Check sheet for the modelled part. Datum: model origin and axes. Units: mm. A direction names the side the tool comes from. Round coordinates to 2 decimals unless told otherwise and drop trailing zeros. Write each loop counter-clockwise with the first axis right and the second up, starting at its lowest first coordinate (ties: lowest second). Pieces come first, ordered by that corner, then holes.
from build123d import *

# Parameters (mm, degrees)
F0_R     = 3.96875
F1_DEPTH = 25.4
F2_R     = 1.524


with BuildPart() as f1:
    # F0 (on Front) → F1 (new body)
    with BuildSketch(Plane.XZ):
        with BuildLine():
            Line((0, 596.9), (0, 0))
            Line((0, 0), (25.4, 0))
            Line((25.4, 0), (25.4, 596.9))
            ThreePointArc((25.4, 596.9), (55.157951, 668.742049), (127, 698.5))
            Line((127, 698.5), (396.875, 698.5))
            Line((396.875, 698.5), (396.875, 723.9))
            Line((396.875, 723.9), (127, 723.9))
            ThreePointArc((127, 723.9), (37.197439, 686.702561), (0, 596.9))
        make_face()
        with Locations((12.7, 120.65)):
            Circle(F0_R, mode=Mode.SUBTRACT)
        with Locations((12.7, 215.9)):
            Circle(F0_R, mode=Mode.SUBTRACT)
    extrude(amount=F1_DEPTH)

    # F2
    f2_edges = [f1.edges().sort_by_distance(p)[0] for p in [
        (25.4, -25.4, 298.45),
        (0, -25.4, 298.45),
        (0, 0, 298.45),
        (25.4, 0, 298.45),
        (12.7, 0, 0),
        (55.157951, 0, 668.742049),
        (261.9375, 0, 698.5),
        (396.875, 0, 711.2),
        (261.9375, 0, 723.9),
        (37.197439, 0, 686.702561),
        (8.73125, 0, 120.65),
        (8.73125, 0, 215.9),
        (12.7, -25.4, 0),
        (55.157951, -25.4, 668.742049),
        (261.9375, -25.4, 698.5),
        (396.875, -25.4, 711.2),
        (261.9375, -25.4, 723.9),
        (37.197439, -25.4, 686.702561),
        (8.73125, -25.4, 120.65),
        (8.73125, -25.4, 215.9),
    ]]
    fillet(f2_edges, radius=F2_R)


solid = f1.part
1. Sectioned sample at C-C, the plane x = 251. Enter the section's corners in (y, z).
2. Set-up check for faces 4 (the cylindrical face through (38.19, -12.544, 687.685)), 5 (the flat face through (25.4, -13, 294)): record each of +Z, -Z, +X, -X, +Y, -Y from which the full face is reachable in a straight line by a thin tool's end or side.
3. Scan lines: line 1 along Z through (x, y) = (12.7, -14.25); line 2 along X through (y, z) = (-15.75, 509.5); line 3 along Z through (x, y) = (200.5, -19.75). Record each from-to range of solid material in increasing order.
4. Release check for a two-part mould opening along Y. For faces 1 (the flat face through (22, 0, 470)), 2 (the flat face through (264, -13, 723.9)), 3 (the flat face through (22, -25.4, 470)) record: released by +Y, released by -Y, zero draft, split by the parting line, or undercut.
5. Go/stop test with flat-tipped pins: pin 1 (5 mm diameter, centred on x = 110, y = -17, fed in from +Z); pin 2 (8 mm diameter, centred on x = 211.5, y = -16, fed in from -Z); pin 3 (6.5 mm diameter, centred on y = -10.5, z = 316, fed in from +X). Record where each tip stops, or that it passes through.
6. Sectioned sample at B-B, the plane z = 547. Enter the section's corners in (x, y), plus the area to 3 significant figures.
7. Sectioned sample at A-A, the plane y = -12.75. Give the number of separate pieces and of enclosed holes in the cut face, plus the area to 3 significant figures.
Computed values:
1. outline: (-25.4, 700.02) arc R1.52 ccw to (-23.88, 698.5) - (-1.52, 698.5) arc R1.52 ccw to (0, 700.02) - (0, 722.38) arc R1.52 ccw to (-1.52, 723.9) - (-23.88, 723.9) arc R1.52 ccw to (-25.4, 722.38) - close
2. face 4: +Z, -X, +Y, -Y
2. face 5: -Z, +X, +Y, -Y
3. line 1: z = 0 to 116.68, 124.62 to 211.93, 219.87 to 652.26
3. line 2: x = 0 to 25.4
3. line 3: z = 698.5 to 723.9
4. face 1: released by +Y
4. face 2: zero draft
4. face 3: released by -Y
5. pin 1: stops at z = 723.07
5. pin 2: stops at z = 698.5
5. pin 3: stops at x = 25.4
6. outline: (0, -23.88) arc R1.52 ccw to (1.52, -25.4) - (23.88, -25.4) arc R1.52 ccw to (25.4, -23.88) - (25.4, -1.52) arc R1.52 ccw to (23.88, 0) - (1.52, 0) arc R1.52 ccw to (0, -1.52) - close
6. area: 643 mm2
7. separate pieces: 1
7. enclosed holes: 2
7. area: 26,500 mm2
